Read the model definition and answer for the solid it produces. Units are mm, in the model's axes. A direction names the side the tool comes from. Give positions to 0.01 mm unless a question says otherwise; leave off trailing zeros. Order: outer loops, then holes, each group sorted by start corner. A loop starts at its lowest first (then second) coordinate and runs counter-clockwise, first axis right, second up. Notation, with made-up numbers: (49, 32) - (60, 32) arc R25 ccw to (60, 56) - close; hole circle Ø7 at (67.25, 64.5). An arc over 180 degrees is marked (long way). Return JSON: item names as keys, results as strings.
```python
from build123d import *

# Parameters (mm, degrees)
SKETCH1_R           = 3.175
SKETCH1_R_2         = 3.174951128
BOSS_EXTRUDE1_DEPTH = 5.842
FILLET2_R           = 12.7
FILLET3_R           = 6.35
CUT_EXTRUDE1_DEPTH  = 87.813654174
BOSS_EXTRUDE2_START = -5.842
BOSS_EXTRUDE2_DEPTH = 5.842
FILLET4_R           = 6.35
SKETCH5_W           = 5.842
SKETCH5_H           = 12.7
SKETCH5_R           = 3.175
BOSS_EXTRUDE3_DEPTH = 5.842
FILLET5_R           = 3.175
FILLET6_R           = 12.7
CUT_EXTRUDE3_DEPTH  = 136.823266385
FILLET7_R           = 3.175
SKETCH8_W           = 15.24
SKETCH8_H           = 4.7625
CUT_EXTRUDE4_DEPTH  = 136.823266529
FILLET8_R           = 1.5875


with BuildPart() as part:
    # Sketch1 → Boss-Extrude1 (new body)
    with BuildSketch(Plane.XY):
        with BuildLine():
            Line((0, 0), (-51.530803591, 0))
            Line((-51.530803591, 0), (-80.587958697, 19.05))
            Line((-80.587958697, 19.05), (-80.587958697, 25.4))
            ThreePointArc((-80.587958697, 25.4), (-74.237958697, 31.75), (-67.887958697, 25.4))
            Line((-67.887958697, 25.4), (-63.5, 25.4))
            Line((-63.5, 25.4), (-11.753958697, 25.4))
            Line((-11.753958697, 25.4), (-0.97772826, 31.02846642))
            ThreePointArc((-0.97772826, 31.02846642), (5.252518949, 30.830896444), (8.311992431, 25.4))
            Line((8.311992431, 25.4), (8.311992431, 0))
            Line((8.311992431, 0), (1.962041303, 0))
            Line((1.962041303, 0), (0, 0))
        make_face()
        with Locations((-74.237958697, 25.4)):
            Circle(SKETCH1_R, mode=Mode.SUBTRACT)
        with Locations((1.962041303, 25.4)):
            Circle(SKETCH1_R_2, mode=Mode.SUBTRACT)
        with BuildLine():
            Line((-17.397521197, 18.95), (-11.952396197, 18.95))
            ThreePointArc((-11.952396197, 18.95), (-11.613642195, 19.090316502), (-11.753958697, 18.7515625))
            Line((-11.753958697, 18.7515625), (-11.753958697, 6.6484375))
            ThreePointArc((-11.753958697, 6.6484375), (-11.613642195, 6.309683498), (-11.952396197, 6.45))
            Line((-11.952396197, 6.45), (-17.397521197, 6.45))
            ThreePointArc((-17.397521197, 6.45), (-17.736275199, 6.309683498), (-17.595958697, 6.6484375))
            Line((-17.595958697, 6.6484375), (-17.595958697, 18.7515625))
            ThreePointArc((-17.595958697, 18.7515625), (-17.736275199, 19.090316502), (-17.397521197, 18.95))
        make_face(mode=Mode.SUBTRACT)
        with BuildLine():
            Line((-43.194396197, 18.95), (-48.639521197, 18.95))
            ThreePointArc((-48.639521197, 18.95), (-48.978275199, 19.090316502), (-48.837958697, 18.7515625))
            Line((-48.837958697, 18.7515625), (-48.837958697, 6.6484375))
            ThreePointArc((-48.837958697, 6.6484375), (-48.978275199, 6.309683498), (-48.639521197, 6.45))
            Line((-48.639521197, 6.45), (-43.194396197, 6.45))
            ThreePointArc((-43.194396197, 6.45), (-42.855642195, 6.309683498), (-42.995958697, 6.6484375))
            Line((-42.995958697, 6.6484375), (-42.995958697, 18.7515625))
            ThreePointArc((-42.995958697, 18.7515625), (-42.855642195, 19.090316502), (-43.194396197, 18.95))
        make_face(mode=Mode.SUBTRACT)
    extrude(amount=BOSS_EXTRUDE1_DEPTH)

    # Fillet2
    # the kernel refuses this fillet: 12.7 mm, written as the material it takes off along each edge
    with BuildSketch(Plane(origin=(-51.530803591, 0, -9.479879108), x_dir=(1, 0, 0), z_dir=(0, 0, 1))) as fillet2_piece_1:
        with BuildLine():
            CenterArc((FILLET2_R * 0.298578869541, FILLET2_R), FILLET2_R, 236.750973169, 33.249026831)
            Line((-FILLET2_R * 0.249700155583, FILLET2_R * 0.163704531514), (0, 0))
            Line((0, 0), (FILLET2_R * 0.298578869541, 0))
        make_face()
    extrude(amount=24.801758216, mode=Mode.SUBTRACT)
    with BuildSketch(Plane(origin=(-80.587958697, 19.05, -17.118170795), x_dir=(0, 1, 0), z_dir=(0, 0, 1))) as fillet2_piece_2:
        with BuildLine():
            CenterArc((6.866738852, -12.689483085), FILLET2_R, 92.331900044, 54.419073124)
            Line((-3.754213598, -5.726339466), (0, 0))
            Line((0, 0), (6.35, 0))
        make_face()
    extrude(amount=40.078341589, mode=Mode.SUBTRACT)

    # Fillet3
    fillet3_edges = [part.edges().sort_by_distance(p)[0] for p in [
        (-67.887958697, 25.4, 2.921),
    ]]
    fillet(fillet3_edges, radius=FILLET3_R)

    # Sketch2 → Cut-Extrude1 (cut, through all)
    with BuildSketch(Plane.XY.offset(5.842)):
        with BuildLine():
            Line((-4.388007569, 5.6435625), (-4.388007569, 0))
            Line((-4.388007569, 0), (8.311992431, 0))
            Line((8.311992431, 0), (8.311992431, 5.6435625))
            Line((8.311992431, 5.6435625), (8.311992431, 5.842))
            Line((8.311992431, 5.842), (8.113554931, 5.842))
            Line((8.113554931, 5.842), (3.739992431, 5.842))
            Line((3.739992431, 5.842), (3.739992431, 9.017))
            Line((3.739992431, 9.017), (6.385358807, 9.017))
            Line((6.385358807, 9.017), (6.385358807, 11.795125))
            Line((6.385358807, 11.795125), (3.739992431, 11.795125))
            Line((3.739992431, 11.795125), (3.739992431, 13.49375))
            Line((3.739992431, 13.49375), (0.183992431, 13.49375))
            Line((0.183992431, 13.49375), (0.183992431, 11.795125))
            Line((0.183992431, 11.795125), (-2.461373945, 11.795125))
            Line((-2.461373945, 11.795125), (-2.461373945, 9.017))
            Line((-2.461373945, 9.017), (0.183992431, 9.017))
            Line((0.183992431, 9.017), (0.183992431, 5.842))
            Line((0.183992431, 5.842), (-4.189570069, 5.842))
            ThreePointArc((-4.189570069, 5.842), (-4.528324071, 5.982316502), (-4.388007569, 5.6435625))
        make_face()
        with BuildLine():
            Line((-36.138007569, 0), (-23.438007569, 0))
            Line((-23.438007569, 0), (-23.438007569, 5.6435625))
            ThreePointArc((-23.438007569, 5.6435625), (-23.297691068, 5.982316502), (-23.636445069, 5.842))
            Line((-23.636445069, 5.842), (-28.010007569, 5.842))
            Line((-28.010007569, 5.842), (-28.010007569, 9.017))
            Line((-28.010007569, 9.017), (-25.364641193, 9.017))
            Line((-25.364641193, 9.017), (-25.364641193, 11.795125))
            Line((-25.364641193, 11.795125), (-28.010007569, 11.795125))
            Line((-28.010007569, 11.795125), (-28.010007569, 13.49375))
            Line((-28.010007569, 13.49375), (-31.566007569, 13.49375))
            Line((-31.566007569, 13.49375), (-31.566007569, 11.795125))
            Line((-31.566007569, 11.795125), (-34.211373945, 11.795125))
            Line((-34.211373945, 11.795125), (-34.211373945, 9.017))
            Line((-34.211373945, 9.017), (-31.566007569, 9.017))
            Line((-31.566007569, 9.017), (-31.566007569, 5.842))
            Line((-31.566007569, 5.842), (-35.939570069, 5.842))
            ThreePointArc((-35.939570069, 5.842), (-36.278324071, 5.982316502), (-36.138007569, 5.6435625))
            Line((-36.138007569, 5.6435625), (-36.138007569, 0))
        make_face()
    extrude(amount=-CUT_EXTRUDE1_DEPTH, mode=Mode.SUBTRACT)

    # Sketch4 → Boss-Extrude2 (add)
    with BuildSketch(Plane.XY.offset(5.842).offset(BOSS_EXTRUDE2_START)):
        with BuildLine():
            Line((-0.97772826, 31.02846642), (-6.365843478, 28.21423321))
            Line((-6.365843478, 28.21423321), (-6.365843478, 76.2))
            Line((-6.365843478, 76.2), (11.486992431, 76.2))
            Line((11.486992431, 76.2), (11.486992431, 0))
            Line((11.486992431, 0), (8.311992431, 0))
            Line((8.311992431, 0), (8.311992431, 5.842))
            Line((8.311992431, 5.842), (8.311992431, 25.4))
            ThreePointArc((8.311992431, 25.4), (5.252518949, 30.830896444), (-0.97772826, 31.02846642))
        make_face()
    extrude(amount=BOSS_EXTRUDE2_DEPTH)

    # Fillet4
    fillet4_edges = [part.edges().sort_by_distance(p)[0] for p in [
        (-6.365843478, 28.21423321, 2.921),
    ]]
    fillet(fillet4_edges, radius=FILLET4_R)

    # Sketch5 → Boss-Extrude3 (add)
    with BuildSketch(Plane.XY.offset(5.842)):
        with BuildLine():
            Line((-50.815843478, 64.726058), (-6.365843478, 64.726058))
            Line((-6.365843478, 64.726058), (-6.365843478, 76.2))
            Line((-6.365843478, 76.2), (11.486992431, 76.2))
            Line((11.486992431, 76.2), (17.306484627, 101.397085752))
            ThreePointArc((17.306484627, 101.397085752), (15.017966748, 107.838377654), (8.211562687, 108.471164514))
            Line((8.211562687, 108.471164514), (-13.583990818, 97.244271998))
            Line((-13.583990818, 97.244271998), (-58.033990818, 97.244271998))
            Line((-58.033990818, 97.244271998), (-66.669907848, 107.028189421))
            ThreePointArc((-66.669907848, 107.028189421), (-74.65021795, 108.299341472), (-77.416513897, 100.706661867))
            Line((-77.416513897, 100.706661867), (-50.815843478, 64.726058))
        make_face()
        with Locations((-45.776642195, 77.426058)):
            Rectangle(SKETCH5_W, SKETCH5_H, mode=Mode.SUBTRACT)
        with Locations((-71.430642195, 102.826058)):
            Circle(SKETCH5_R, mode=Mode.SUBTRACT)
        with Locations((-14.873396197, 77.426058)):
            Rectangle(SKETCH5_W, SKETCH5_H, mode=Mode.SUBTRACT)
        with Locations((11.119357805, 102.826058)):
            Circle(SKETCH5_R, mode=Mode.SUBTRACT)
    extrude(amount=-BOSS_EXTRUDE3_DEPTH)

    # Fillet5
    fillet5_edges = [part.edges().sort_by_distance(p)[0] for p in [
        (-6.365843478, 64.726058, 2.921),
    ]]
    fillet(fillet5_edges, radius=FILLET5_R)

    # Fillet6
    fillet6_edges = [part.edges().sort_by_distance(p)[0] for p in [
        (11.486992431, 76.2, 2.921),
        (-50.815843478, 64.726058, 2.921),
        (-58.033990818, 97.244271998, 2.921),
        (-13.583990818, 97.244271998, 2.921),
    ]]
    fillet(fillet6_edges, radius=FILLET6_R)

    # Sketch7 → Cut-Extrude3 (cut, through all)
    with BuildSketch(Plane.XY.offset(5.842)):
        with BuildLine():
            Line((8.311992431, 71.577463591), (8.311992431, 41.414963591))
            ThreePointArc((8.311992431, 41.414963591), (9.2419284, 39.16989956), (11.486992431, 38.239963591))
            Line((11.486992431, 38.239963591), (11.486992431, 74.752463591))
            ThreePointArc((11.486992431, 74.752463591), (9.2419284, 73.822527621), (8.311992431, 71.577463591))
        make_face()
    extrude(amount=-CUT_EXTRUDE3_DEPTH, mode=Mode.SUBTRACT)

    # Fillet7
    fillet7_edges = [part.edges().sort_by_distance(p)[0] for p in [
        (11.486992431, 74.752463591, 2.921),
        (11.486992431, 38.239963591, 2.921),
    ]]
    fillet(fillet7_edges, radius=FILLET7_R)

    # Sketch8 → Cut-Extrude4 (cut, through all)
    with BuildSketch(Plane.XY.offset(5.842)):
        with Locations((-30.155642195, 80.639021998)):
            Rectangle(SKETCH8_W, SKETCH8_H)
        with Locations((-30.155642195, 88.513021998)):
            Rectangle(SKETCH8_W, SKETCH8_H)
        with Locations((-30.155642195, 72.765021998)):
            Rectangle(SKETCH8_W, SKETCH8_H)
    extrude(amount=-CUT_EXTRUDE4_DEPTH, mode=Mode.SUBTRACT)

    # Fillet8
    fillet8_edges = [part.edges().sort_by_distance(p)[0] for p in [
        (-37.775642195, 86.131771998, 2.921),
        (-37.775642195, 90.894271998, 2.921),
        (-22.535642195, 90.894271998, 2.921),
        (-22.535642195, 86.131771998, 2.921),
        (-22.535642195, 78.257771998, 2.921),
        (-37.775642195, 78.257771998, 2.921),
        (-37.775642195, 83.020271998, 2.921),
        (-22.535642195, 83.020271998, 2.921),
        (-22.535642195, 70.383771998, 2.921),
        (-37.775642195, 70.383771998, 2.921),
        (-37.775642195, 75.146271998, 2.921),
        (-22.535642195, 75.146271998, 2.921),
    ]]
    fillet(fillet8_edges, radius=FILLET8_R)


solid = part.part
```
Q1. Given pin 1 (5.5 mm diameter, centred on x = -74.24, y = 25.4, fed in from +Z); pin 2 (2.5 mm diameter, centred on y = 7, z = 2.5, fed in from -X); pin 3 (2 mm diameter, centred on x = 5, z = 3, fed in from -Y); pin 4 (1.8 mm diameter, centred on y = 10.5, z = 2, fed in from +X), each flat-ended and moving along its own axis, determine where each tip first touches the part or whether it passes through.
Values:
{"pin 1": "passes through", "pin 2": "stops at x = -64.11", "pin 3": "stops at y = 5.84", "pin 4": "stops at x = 11.49"}
Q2. Determine the mould class of faces 1 (the flat face through (-34, 97.244, 3)), 2 (the cylindrical face through (8.777, 73.232, 2.962)), 3 (the flat face through (-66.18, 85.51, 2.96)) for opening direction X: released by +X, released by -X, zero draft, split by the parting line, or undercut.
Values:
{"face 1": "undercut", "face 2": "released by +X", "face 3": "released by -X"}
Q3. A cutting plane is placed at C-C (y = 95). Write down the section's boundary in (x, z).
Values:
{"outline": "(-73.2, 0) - (15.83, 0) - (15.83, 5.84) - (-73.2, 5.84) - close"}
Q4. A cutting plane is placed at B-B (z = 4.2). Give the number of separate pieces and of enclosed holes in the cut face, and give its area (3 significant figures).
Values:
{"separate pieces": "1", "enclosed holes": "11", "area": "4,700 mm²"}
Q5. For faces 4 (the flat face through (-30, 70.384, 3)), 5 (the flat face through (-21, 67, 0)), 6 (the flat face through (-34, 5.842, 3)), determine the directions among +Z, -Z, +X, -X, +Y, -Y from which every point of the face is accessible in a straight line to the end or side of a thin tool.
Values:
{"face 4": "+Z, -Z", "face 5": "-Z, +X, -X, +Y, -Y", "face 6": "+Z, -Z, -Y"}
Q6. A cutting plane is placed at A-A (y = 58). Write down the section's boundary in (x, z), and give its area (3 significant figures).
Values:
{"outline": "(-6.37, 0) - (8.31, 0) - (8.31, 5.84) - (-6.37, 5.84) - close", "area": "85.7 mm²"}
Q7. Consider L1, parallel to X at y = 17.5, z = 3.95; L2, parallel to Y at x = -30, z = 3.2; L3, parallel to Y at x = -26.5, z = 3.2. Determine where each line is inside the solid, lowest interval first.
Values:
{"L1": "x = -77.41 to -48.84, -43 to -17.6, -11.75 to 11.49", "L2": "y = 13.49 to 25.4, 64.73 to 70.38, 75.15 to 78.26, 83.02 to 86.13, 90.89 to 97.24", "L3": "y = 5.84 to 9.02, 11.8 to 25.4, 64.73 to 70.38, 75.15 to 78.26, 83.02 to 86.13, 90.89 to 97.24"}
